from build123d import *

# Parameters (mm, degrees)
EXTRUDE_1_DEPTH     = 220
SKETCH_2_R          = 4.25
CUT_EXTRUDE_1_DEPTH = 2


with BuildPart() as part:
    # Эскиз1 → Бобышка-Вытянуть1 (new body)
    with BuildSketch(Plane(origin=(0, 0, 0), x_dir=(1, 0, 0), z_dir=(0, 1, 0))):
        Polygon((0, 0), (0, 20), (1, 20), (1, 1), (20, 1), (20, 0), align=None)
    extrude(amount=EXTRUDE_1_DEPTH)

    # Эскиз2 → Вырез-Вытянуть1 (cut, through all)
    with BuildSketch(Plane(origin=(1, 0, 0), x_dir=(0, 0, -1), z_dir=(1, 0, 0))):
        with Locations((10.5, 180)):
            Circle(SKETCH_2_R)
        with Locations((10.5, 110)):
            Circle(SKETCH_2_R)
        with Locations((10.5, 40)):
            Circle(SKETCH_2_R)
    extrude(amount=-CUT_EXTRUDE_1_DEPTH, mode=Mode.SUBTRACT)


solid = part.part
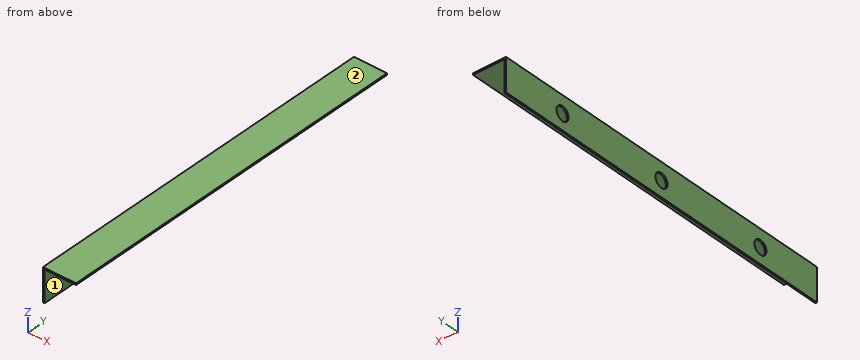
Geometry check sheet. Reference: the model listing, model coordinates, mm. Face numbers are marked on the shaded views. A direction names the side the tool comes from. Give positions to 0.01 mm unless a question says otherwise; leave off trailing zeros. Write each loop counter-clockwise with the first axis right and the second up, starting at its lowest first coordinate (ties: lowest second). Pieces come first, ordered by that corner, then holes.
1) Set-up check for the marked faces 1 and 2: record each of +Z, -Z, +X, -X, +Y, -Y from which the full face is reachable in a straight line by a thin tool's end or side.
Values follow:
face 1: -Z, +X, +Y, -Y
face 2: +Z, +X, -X, +Y, -Y
2) Go/stop test with flat-tipped pins: pin 1 Ø2 at (y, z) = (112.5, -10.5) entering from +X; pin 2 Ø1 at (x, y) = (9, 146.5) entering from -Z; pin 3 Ø3 at (y, z) = (39.5, -6.5) entering from +X. Record where each tip stops, or that it passes through.
Values follow:
pin 1: passes through
pin 2: stops at z = -1
pin 3: stops at x = 1
3) Thickness scan on line 1 (Y direction, x = 0.4, z = -10.5); line 2 (X direction, y = 190, z = -8.25); line 3 (Z direction, x = 16, y = 206). Record the ranges inside material, lowest first.
Values follow:
line 1: y = 0 to 35.75, 44.25 to 105.75, 114.25 to 175.75, 184.25 to 220
line 2: x = 0 to 1
line 3: z = -1 to 0
4) Cross-section at A-A (z = -12.5). Record the boundary of the cut face in (x, y).
Values follow:
outline: (0, 0) - (1, 0) - (1, 36.25) - (0, 36.25) - close; (0, 43.75) - (1, 43.75) - (1, 106.25) - (0, 106.25) - close; (0, 113.75) - (1, 113.75) - (1, 176.25) - (0, 176.25) - close; (0, 183.75) - (1, 183.75) - (1, 220) - (0, 220) - close
5) Cross-section at B-B (y = 110). Record the boundary of the cut face in (x, z), plus the area to 3 significant figures.
Values follow:
outline: (0, -20) - (1, -20) - (1, -14.75) - (0, -14.75) - close; (0, -6.25) - (1, -6.25) - (1, -1) - (20, -1) - (20, 0) - (0, 0) - close
area: 30.5 mm2
6) Cross-section at D-D (x = 11.5). Record the boundary of the cut face in (y, z).
Values follow:
outline: (0, -1) - (220, -1) - (220, 0) - (0, 0) - close
7) Cross-section at C-C (y = 58). Record the boundary of the cut face in (x, z).
Values follow:
outline: (0, -20) - (1, -20) - (1, -1) - (20, -1) - (20, 0) - (0, 0) - close
